from build123d import *

# Parameters (mm, degrees)
FILLET1_R = 0.5


with BuildPart() as part:
    # Sketch1 → Revolve1 (revolve)
    with BuildSketch(Plane.XY):
        with BuildLine():
            Line((1.677050983, 6.5), (3.5, 6.5))
            Line((3.5, 6.5), (3.5, 5))
            Line((3.5, 5), (-3.5, 5))
            Line((-3.5, 5), (-3.5, 6.5))
            Line((-3.5, 6.5), (-1.677050983, 6.5))
            ThreePointArc((-1.677050983, 6.5), (0, 5.75), (1.677050983, 6.5))
        make_face()
    revolve(axis=Axis((-42.390929705, 0, 0), (1, 0, 0)))

    # Fillet1
    fillet1_edges = [part.edges().sort_by_distance(p)[0] for p in [
        (3.5, -5, 0),
        (-3.5, -5, 0),
    ]]
    fillet(fillet1_edges, radius=FILLET1_R)


solid = part.part
Build history of the part. All positions in model axes, mm. Round coordinates to 2 decimals unless told otherwise and drop trailing zeros. Write each loop counter-clockwise with the first axis right and the second up, starting at its lowest first coordinate (ties: lowest second). Pieces come first, ordered by that corner, then holes. Notation, with made-up numbers: (54.25, 30) - (85.25, 30) arc R17 ccw to (85.25, 42) - close; hole circle Ø3 at (-30, 75). An arc over 180 degrees is marked (long way). Use CSV: the item, a comma, the result in double quotes.
(1) Mould opens along Y. For faces 1 (the cylindrical face through (-2.576, -5.158, -3.955)), 2 (the cylindrical face through (-0.04, -1.08, -4.88)), 3 (the flat face through (3.5, -5, 3)) say: pulls with the +Y half, pulls with the -Y half, needs draft (parallel to the pull), parting line crosses it, or undercut.
Response:
face 1,"parting line crosses it"
face 2,"undercut"
face 3,"needs draft"
(2) Wall check: line 1 (Z direction, x = 1, y = -2.5); line 2 (X direction, y = -3.25, z = -5.5); line 3 (Y direction, x = 1.5, z = -3). Give the ranges that are in metal, low to high.
Response:
line 1,"-5.44 to -4.33, 4.33 to 5.44"
line 2,"-3.5 to -1.57, 1.57 to 3.5"
line 3,"-5.57 to -4, 4 to 5.57"
(3) Pin check, flat tips, straight feed: P1, Ø2, axis at x = 2.5, y = 2.5, coming from the -Z side; P2, Ø6, axis at y = 0, z = 0, coming from the -X side. Stop position of each tip, or through.
Response:
P1,"z = -6.32"
P2,"through"
(4) Band-saw the part on C-C (x = -2). Write the cut outline in (y, z).
Response:
outline,"circle Ø13 at (0, 0); hole circle Ø10 at (0, 0)"
(5) Band-saw the part on A-A (z = 0). Write the cut outline in (x, y).
Response:
outline,"(-3.5, -6.5) - (-1.68, -6.5) arc R2.25 cw to (1.68, -6.5) - (3.5, -6.5) - (3.5, -5.5) arc R0.5 ccw to (3, -5) - (-3, -5) arc R0.5 ccw to (-3.5, -5.5) - close; (-3.5, 5.5) arc R0.5 ccw to (-3, 5) - (3, 5) arc R0.5 ccw to (3.5, 5.5) - (3.5, 6.5) - (1.68, 6.5) arc R2.25 cw to (-1.68, 6.5) - (-3.5, 6.5) - close"
(6) Band-saw the part on D-D (x = -0.25). Write the cut outline in (y, z).
Response:
outline,"circle Ø11.53 at (0, 0); hole circle Ø10 at (0, 0)"
